Read the model definition and answer for the solid it produces. Units are mm, in the model's axes. Coordinates: 2 decimals unless noted, no trailing zeros. Order: outer loops, then holes, each group sorted by start corner. A loop starts at its lowest first (then second) coordinate and runs counter-clockwise, first axis right, second up. Notation, with made-up numbers: M 78,68 L 86,68 A20 ccw 86,86 Z; hole C -17,61 d1. An arc over 180 degrees is marked long. Put each result on its own line as item: value.
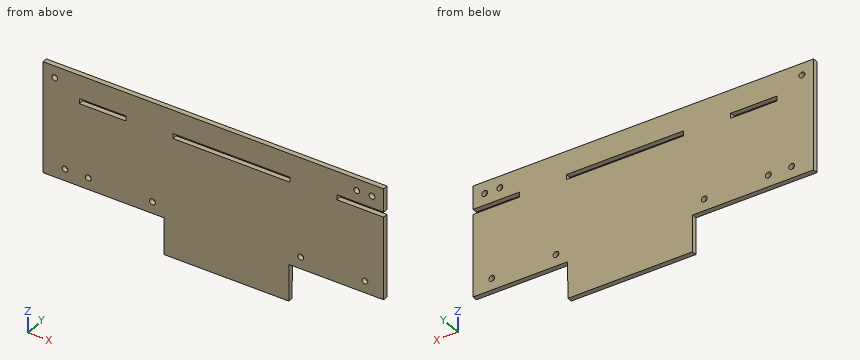
from build123d import *

# Parameters (mm, degrees)
SKETCH1_W           = 50.6476
SKETCH1_H           = 5.4102
SKETCH1_R           = 3.175
BOSS_EXTRUDE1_DEPTH = 5.4102
BOSS_EXTRUDE3_DEPTH = 5.4102


with BuildPart() as part:
    # Sketch1 → Boss-Extrude1 (new body)
    with BuildSketch(Plane(origin=(0, 0, 0), x_dir=(1, 0, 0), z_dir=(0, 1, 0))):
        Polygon((-205.105, 47.5361), (-205.105, -72.9361), (165.481, -72.9361), (165.481, -47.5361), (114.8334, -47.5361), (114.8334, -42.1259), (165.481, -42.1259), (165.481, 47.5361), (62.5475, 47.5361), (62.5475, -42.1259), (63.7286, -42.1259), (63.7286, -47.5361), (-63.7286, -47.5361), (-63.7286, -42.1259), (-73.30694, -42.1259), (-73.30694, 47.5361), align=None)
        with Locations((-140.1572, -44.831)):
            Rectangle(SKETCH1_W, SKETCH1_H, mode=Mode.SUBTRACT)
        with Locations(Location((-181.229, 34.8361, 0), (0, 0, 270))):
            Circle(SKETCH1_R, mode=Mode.SUBTRACT)
        with Locations(Location((152.781, -60.2361, 0), (0, 0, 270))):
            Circle(SKETCH1_R, mode=Mode.SUBTRACT)
        with Locations(Location((-192.405, -60.2361, 0), (0, 0, 270))):
            Circle(SKETCH1_R, mode=Mode.SUBTRACT)
        with Locations(Location((136.271, -60.2361, 0), (0, 0, 270))):
            Circle(SKETCH1_R, mode=Mode.SUBTRACT)
        with Locations(Location((-155.829, 34.8361, 0), (0, 0, 270))):
            Circle(SKETCH1_R, mode=Mode.SUBTRACT)
        with Locations(Location((-86.00694, 34.8361, 0), (0, 0, 270))):
            Circle(SKETCH1_R, mode=Mode.SUBTRACT)
        with Locations(Location((145.06956, 34.8361, 0), (0, 0, 270))):
            Circle(SKETCH1_R, mode=Mode.SUBTRACT)
        with Locations(Location((75.2475, 34.8361, 0), (0, 0, 270))):
            Circle(SKETCH1_R, mode=Mode.SUBTRACT)
    extrude(amount=BOSS_EXTRUDE1_DEPTH)

    # Sketch2 → Boss-Extrude3 (add)
    with BuildSketch(Plane(origin=(0, 5.4102, 0), x_dir=(1, 0, 0), z_dir=(0, 1, 0))):
        Polygon((-63.7286, -42.1259), (62.5475, -42.1259), (62.5475, 47.5361), (62.280495402, 87.4141), (-73.30694, 87.4141), (-73.30694, 47.5361), (-73.30694, -42.1259), align=None)
    extrude(amount=-BOSS_EXTRUDE3_DEPTH)


solid = part.part
Q1. Find section D-D on z = -61. Write down the section's boundary in (x, y), plus the area to 3 significant figures.
Answers below:
outline: M -73.31,0 L 62.46,0 L 62.46,5.41 L -73.31,5.41 Z
area: 735 mm^2
Q2. Find section B-B on y = 4.2. Give the number of separate pieces and of enclosed holes in the cut face, plus the area to 3 significant figures.
Answers below:
separate pieces: 1
enclosed holes: 10
area: 48,600 mm^2
Q3. Find section C-C on x = 19.5. Write down the section's boundary in (y, z), plus the area to 3 significant figures.
Answers below:
outline: M 0,-87.41 L 5.41,-87.41 L 5.41,42.13 L 0,42.13 Z; M 0,47.54 L 5.41,47.54 L 5.41,72.94 L 0,72.94 Z
area: 838 mm^2
Q4. Given pin 1 (2.5 mm diameter, centred on x = -148, y = 2.5, fed in from -Z); pin 2 (2.5 mm diameter, centred on y = 2, z = -69, fed in from -X); pin 3 (2.5 mm diameter, centred on y = 3.5, z = 44.5, fed in from +X), each flat-ended and moving along its own axis, determine where each tip first touches the part or whether it passes through.
Answers below:
pin 1: stops at z = -47.54
pin 2: stops at x = -73.31
pin 3: stops at x = 114.83
Q5. Consider line 1 along X through (y, z) = (1.45, 44.5) (3 decimals); line 2 along Z through (x, y) = (-156, 2.95); line 3 along Z through (x, y) = (-151.5, 4.6). Determine where each line is inside the solid, lowest interval first.
Answers below:
line 1: x = -205.105 to -165.481, -114.833 to -63.729, 63.729 to 114.833
line 2: z = -47.54 to -38.01, -31.67 to 42.13, 47.54 to 72.94
line 3: z = -47.54 to 42.13, 47.54 to 72.94
Q6. Find section A-A on x = 119.5. Write down the section's boundary in (y, z), plus the area to 3 significant figures.
Answers below:
outline: M 0,-47.54 L 5.41,-47.54 L 5.41,42.13 L 0,42.13 Z; M 0,47.54 L 5.41,47.54 L 5.41,72.94 L 0,72.94 Z
area: 623 mm^2
